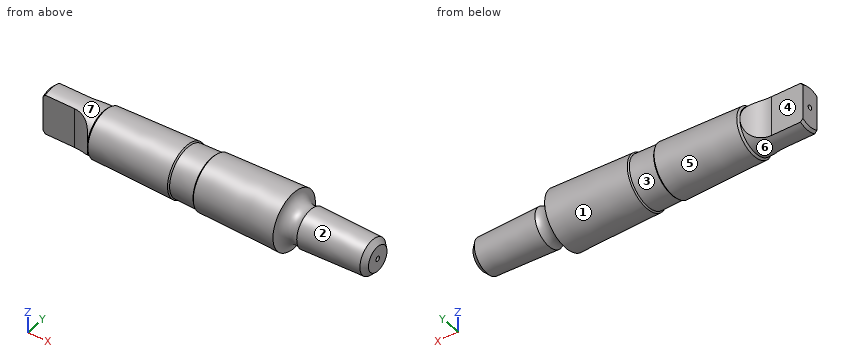
```python
from build123d import *

# Parameters (mm, degrees)
CHANFREIN1_SIZE         = 1
CHANFREIN2_SIZE         = 2
CHANFREIN2_SIZE2        = 2.055782961
ENL_V_MAT_EXTRU_1_DEPTH = 15


with BuildPart() as part:
    # Esquisse1 → Révolution1 (revolve)
    with BuildSketch(Plane.XY, mode=Mode.PRIVATE) as r_volution1_sk:
        with BuildLine():
            Line((-102.251641217, 9.25), (-79.75, 9.25))
            Line((-79.75, 9.25), (-79, 10))
            Line((-79, 10), (-44.998238309, 10.860804093))
            Line((-44.998238309, 10.860804093), (-44.485744289, 10.373618421))
            Line((-44.485744289, 10.373618421), (-34.488947364, 10.626701887))
            Line((-34.488947364, 10.626701887), (-34.001761691, 11.139195907))
            Line((-34.001761691, 11.139195907), (0, 12))
            ThreePointArc((0, 12), (2.339354929, 7.968871126), (7, 8))
            Line((7, 8), (35, 7.25))
            Line((35, 7.25), (35, 1))
            Line((35, 1), (34, 0))
            Line((34, 0), (-101.251641217, 0))
            Line((-101.251641217, 0), (-102.251641217, 1))
            Line((-102.251641217, 1), (-102.251641217, 9.25))
        make_face()
    revolve(r_volution1_sk.sketch.rotate(Axis((0, 0, 0), (1, 0, 0)), 90), axis=Axis((0, 0, 0), (1, 0, 0)))

    # Chanfrein1
    chanfrein1_edges = [part.edges().sort_by_distance(p)[0] for p in [
        (-102.251641217, 0, -9.25),
    ]]
    chamfer(chanfrein1_edges, length=CHANFREIN1_SIZE)

    # Chanfrein2
    chanfrein2_edges = [part.edges().sort_by_distance(p)[0] for p in [
        (35, 0, -7.25),
    ]]
    chanfrein2_side = [part.faces().sort_by_distance(p)[0] for p in [
        (35, 0, -7.044939033),
    ]]
    chamfer(chanfrein2_edges, length=CHANFREIN2_SIZE, length2=CHANFREIN2_SIZE2, reference=chanfrein2_side[0])

    # Esquisse2 → Enlèv. mat.-Extru.1 (cut, symmetric)
    with BuildSketch(Plane.XY):
        with BuildLine():
            Line((-89.127499667, 4), (-102.251641217, 4))
            Line((-102.251641217, 4), (-102.251641217, 16))
            Line((-102.251641217, 16), (-78.127499667, 16))
            Line((-78.127499667, 16), (-78.127499667, 15))
            ThreePointArc((-78.127499667, 15), (-81.349325074, 7.221825407), (-89.127499667, 4))
        make_face()
    enl_v_mat_extru_1 = extrude(amount=ENL_V_MAT_EXTRU_1_DEPTH, both=True, mode=Mode.SUBTRACT)

    # Symétrie1: Enlèv. mat.-Extru.1 across plane
    add(enl_v_mat_extru_1.mirror(Plane.ZX), mode=Mode.SUBTRACT)


solid = part.part
```
For this review, take the finished solid that the model builds, in its own axes (mm). Face numbers are marked on the shaded views. A direction names the side the tool comes from. Coordinates: 2 decimals unless noted, no trailing zeros. Write each loop counter-clockwise with the first axis right and the second up, starting at its lowest first coordinate (ties: lowest second). Pieces come first, ordered by that corner, then holes.
(1) Wall thickness on probe 1 along Y at (x, z) = (-35, -5.25); probe 2 along Y at (x, z) = (-84, -3); probe 3 along Z at (x, y) = (-19.5, 7): over which ranges is each line inside the solid? List them lowest first.
(2) Add section C-C on x = -39. Give the boundary of the cut face in (y, z) (1 decimal).
(3) Add section A-A on x = -84. Give the boundary of the cut face in (y, z), then the cut area to 3 significant figures.
(4) The part is to be moulded in two halves that separate along X. For the marked faces 1, 2 and 3, say which applies: +X half, -X half, draft (parallel to the pull), parting line (faces both ways), or undercut.
(5) For pin 1 Ø6 at (x, z) = (-79, -2) entering from -Y; pin 2 Ø6.5 at (x, z) = (-93, -2) entering from -Y; pin 3 Ø1.5 at (x, y) = (-35.5, 3.5) entering from -Z, all flat-tipped, find the tip position at first contact; note any pin that passes through.
(6) Tool access review of the marked faces 4, 5, 6 and 7: name each direction out of +Z, -Z, +X, -X, +Y, -Y from which nothing blocks a thin tool from reaching the whole face with its end or side.
(7) Add section B-B on x = 19.5. Give the boundary of the cut face in (y, z).
Answer sheet:
1. probe 1: y = -9.22 to 9.22
1. probe 2: y = -5.27 to 5.27
1. probe 3: z = -9.13 to 9.13
2. outline: circle Ø21 at (0, 0)
3. outline: (-5.27, -7.6) arc R9.25 ccw to (5.27, -7.6) - (5.27, 7.6) arc R9.25 ccw to (-5.27, 7.6) - close
3. area: 184 mm2
4. face 1: -X half
4. face 2: +X half
4. face 3: undercut
5. pin 1: stops at y = -10.06
5. pin 2: stops at y = -4
5. pin 3: stops at z = -10.24
6. face 4: +Z, -Z, -X, +Y
6. face 5: -X
6. face 6: -Z, -X
6. face 7: +Z, -X
7. outline: circle Ø15.33 at (0, 0)
